Autodesk Inventor part; units mm, degrees
ref_plane "YZ Plane" through (0, 0, 0) normal (1, 0, 0) x (0, 1, 0)
ref_plane "XZ Plane" through (0, 0, 0) normal (0, 1, 0) x (-1, 0, 0)
ref_plane "XY Plane" through (0, 0, 0) normal (0, 0, 1) x (1, 0, 0)
sketch "Skizze1" plane through (0, 0, 0) normal (0, 0, 1) x (1, 0, 0)
  line L0 (15, 7.5) -> (15, -7.5)
  line L1 (15, -7.5) -> (-15, -7.5)
  line L2 (-15, -7.5) -> (-15, 7.5)
  line L3 (-15, 7.5) -> (15, -7.5) construction
  line L4 (15, 7.5) -> (-15, -7.5) construction
  arc A0 (-12.5, 7.5) -> (13.5, 7.5) centre (0.5, 7.5) ccw
  line L5 (-15, 7.5) -> (-12.5, 7.5)
  line L6 (13.5, 7.5) -> (15, 7.5)
  point P0 (0, 0)
  dimension "d0" = 30
  dimension "d1" = 15
  dimension "d2" = 26
extrude "Extrusion1" add sketch "Skizze1" along normal blind 65
sketch "Skizze2" plane through (0, 0, 65) normal (0, 0, 1) x (1, 0, 0)
  line L0 (-15, 7.5) -> (-15, -7.5)
  line L1 (15, 7.5) -> (13.5, 7.5)
  line L2 (-15, -7.5) -> (15, -7.5)
  line L3 (15, -7.5) -> (15, 7.5)
  line L4 (-15, 7.5) -> (-15, -7.5)
  arc A0 (-12.5, 7.5) -> (13.5, 7.5) centre (0.5, 7.5) ccw
  arc A1 (0, -5.4904) -> (13.5, 7.5) centre (0.5, 7.5) ccw
  arc A2 (-12.5, 7.5) -> (0, -5.4904) centre (0.5, 7.5) ccw
  point P0 (0, 0)
extrude "Extrusion2" [suppressed]
sketch "Skizze3" plane through (0, 0, 67) normal (0, 0, 1) x (1, 0, 0)
  line L0 (-15, 7.5) -> (-15, -7.5)
  line L1 (-15, -7.5) -> (15.179, -7.5)
  line L2 (15.179, -7.5) -> (15.179, 7.5)
  line L3 (15.179, 7.5) -> (-15, 7.5)
  line L4 (-15, 7.5) -> (-15, -7.5)
  arc A0 (-12.9105, 7.5) -> (13.0895, 7.5) centre (0.0895, 7.5) ccw
  point P0 (0, 0)
  dimension "d7" = 26
extrude "Extrusion3" [suppressed]
sketch "Skizze4" plane through (0, 0, 132) normal (0, 0, 1) x (1, 0, 0)
  line L0 (-15, 7.5) -> (-15, -7.5)
  line L1 (-15, -7.5) -> (15, -7.5)
  line L2 (15, -7.5) -> (15, 12.5)
  line L3 (15, 12.5) -> (-15, 12.5)
  line L4 (-15, 12.5) -> (-15, -7.5)
  point P0 (0, 0)
  dimension "d10" = 30
  dimension "d11" = 20
extrude "Extrusion4" [suppressed]
sketch "Skizze5" plane through (0, 0, 134) normal (0, 0, 1) x (1, 0, 0)
  circle A0 centre (0, 7.5) radius 2.5
  point P0 (0, 0)
  dimension "d14" = 5
extrude "Extrusion5" [suppressed]
sketch "Skizze6" plane through (0, 0, 0) normal (0, 0, -1) x (-1, 0, 0)
  line L0 (-15.179, -7.5) -> (-15, -7.5)
  line L1 (-15, 12.5) -> (15, 12.5)
  line L2 (-15, -7.5) -> (15, -7.5)
  line L3 (15, -7.5) -> (15, 12.5)
  line L4 (15, 12.5) -> (-15, 12.5)
  line L5 (-15, 12.5) -> (-15, -7.5)
  point P0 (0, 0)
  point P1 (-14.9426, -7.5)
extrude "Extrusion6" add sketch "Skizze6" along normal blind 2
sketch "Skizze7" plane through (0, 0, -2) normal (0, 0, -1) x (-1, 0, 0)
  line L0 (-13.0895, 7.5) -> (12.9105, 7.5)
  circle A0 centre (0, 7.5) radius 2.5
  point P0 (0, 0)
  dimension "d19" = 5
extrude "Extrusion7" cut sketch "Skizze7" against normal blind 2
fillet "Rundung1" radius 2 1 edges at (-15, 12.5, -1)
fillet "Rundung2" [suppressed]
fillet "Rundung3" [suppressed]
fillet "Rundung4" radius 2 1 edges at (15, 12.5, -1)
sketch "Skizze8" plane through (-15, -7.5, -2) normal (-1, 0, 0) x (0, 0, 1)
  line L0 (69, 0) -> (69, 15)
  line L1 (69, 15) -> (68, 15)
  line L2 (75.5, 13) -> (60.5, 13)
  line L3 (60.5, 13) -> (60.5, 15)
  line L4 (75.5, 15) -> (75.5, 13)
  line L5 (75.5, 13) -> (60.5, 17) construction
  line L6 (60.5, 13) -> (68, 15) construction
  line L7 (2, 15) -> (67, 15)
  line L8 (60.5, 15) -> (75.5, 15)
  point P0 (2, 7.5)
  dimension "d26" = 1
  dimension "d28" = 4
extrude "Extrusion8" add sketch "Skizze8" along normal blind 15
sketch "Skizze9" plane through (-12.5, 7.5, 65) normal (0, 1, 0) x (1, 0, 0)
  line L0 (-2.5, 6.5) -> (-17.5, 6.5)
  line L1 (-2.5, 67) -> (-2.5, 0)
  line L2 (-17.5, 6.5) -> (3.7132, 6.5) construction
  circle A0 centre (-10, -1) radius 2.5
  point P0 (12.5, 65)
  point P1 (-2.5, -69)
  dimension "d32" = 5
extrude "Extrusion9" cut sketch "Skizze9" against normal through all
sketch "Skizze10" plane through (15, -7.5, 67) normal (1, 0, 0) x (0, 0, -1)
  line L0 (0, 15) -> (1, 15)
  line L1 (67, 15) -> (2, 15)
  line L2 (8.5, 17) -> (-6.5, 17)
  line L3 (-6.5, 15) -> (-6.5, 13)
  line L4 (-6.5, 13) -> (8.5, 13)
  line L5 (8.5, 13) -> (8.5, 15)
  line L6 (1, 15) -> (-6.5, 13) construction
  line L7 (1, 15) -> (8.5, 13) construction
  line L8 (0, 15) -> (-65, 15)
  line L9 (-6.5, 15) -> (8.5, 15)
  point P0 (67, 7.5)
  point P1 (8.5, 15)
  point P2 (1, 15)
  dimension "d35" = 1
  dimension "d37" = 4
extrude "Extrusion10" add sketch "Skizze10" along normal blind 15
sketch "Skizze11" plane through (-12.5, 7.5, 65) normal (0, 1, 0) x (1, 0, 0)
  line L0 (27.679, -8.5) -> (27.679, -67)
  line L1 (42.5, -8.5) -> (42.5, 6.5)
  line L2 (27.679, -8.5) -> (48.6391, -8.5) construction
  line L3 (27.5, 6.5) -> (27.5, 0)
  circle A0 centre (35, -1) radius 2.5
  point P0 (12.5, 65)
  point P1 (27.5, -2)
  dimension "d41" = 5
extrude "Extrusion11" cut sketch "Skizze11" against normal through all
properties part number "Motorhalterung"
Design review of the part built by this model. Coordinates are the model's own, in mm. A direction names the side the tool comes from. Round coordinates to 2 decimals unless told otherwise and drop trailing zeros. Write each loop counter-clockwise with the first axis right and the second up, starting at its lowest first coordinate (ties: lowest second). Pieces come first, ordered by that corner, then holes.
Item 1: The part is to be moulded in two halves that separate along X. For faces 1 (the cylindrical face through (-14.43, 11.9, -1.01)), 2 (the flat face through (15, 7, 69)), 3 (the flat face through (20, 7.5, 59)), say which applies: +X half, -X half, draft (parallel to the pull), parting line (faces both ways), or undercut.
Item 2: We need section A-A on x = -22.5. Write out the cut boundary in (y, z), and give its area (3 significant figures).
Item 3: We need section D-D on x = 0. Write out the cut boundary in (y, z), and give its area (3 significant figures).
Item 4: We need section C-C on y = -2. Write out the cut boundary in (x, z).
Item 5: For probe 1 along X at (y, z) = (6.7, 66); probe 2 along Z at (x, y) = (22.5, 6); probe 3 along X at (y, z) = (7.5, -1.2), list the stretches that pass through material, from the lowest coordinate up.
Item 6: Clearance check with flat-ended pins moving along their axes: pin 1 Ø4.5 at (x, y) = (-3.5, -2) entering from +Z; pin 2 Ø3 at (x, y) = (0, 7.5) entering from -Z; pin 3 Ø12 at (x, z) = (-24.5, 62.5) entering from -Y; pin 4 Ø10 at (x, z) = (22, 63.5) entering from +Y. State where each tip first meets the part, or that it passes through.
Item 7: We need section B-B on z = 57.5. Write out the cut boundary in (x, y).
Item 8: For faces 4 (the flat face through (-19, 5.5, 66)), 5 (the flat face through (-22, 6, 58.5)), 6 (the flat face through (19, 5.5, 66)), 7 (the flat face through (-15, 7, 69)), list the 3-axis set-ups (+Z, -Z, +X, -X, +Y, -Y) from which the entire face can be reached by the end or side of a thin tool; tool diameter is ignored.
Returned:
1. face 1: -X half
1. face 2: undercut
1. face 3: draft
2. outline: (5.5, 58.5) - (7.5, 58.5) - (7.5, 63.5) - (5.5, 63.5) - close; (5.5, 68.5) - (7.5, 68.5) - (7.5, 73.5) - (5.5, 73.5) - close
2. area: 20.0 mm2
3. outline: (-7.5, -2) - (5, -2) - (5, 0) - (-5.49, 0) - (-5.49, 65) - (-7.5, 65) - close; (10, -2) - (12.5, -2) - (12.5, 0) - (10, 0) - close
3. area: 161 mm2
4. outline: (-15, -2) - (15, -2) - (15, 65) - (9.37, 65) - (9.37, 0) - (-8.37, 0) - (-8.37, 65) - (-15, 65) - close
5. probe 1: x = -30 to -25, -20 to -15, 15 to 20, 25 to 30
5. probe 2: z = 58.5 to 63.5, 68.5 to 73.5
5. probe 3: x = -15 to -2.5, 2.5 to 15
6. pin 1: stops at z = 0
6. pin 2: passes through
6. pin 3: stops at y = 5.5
6. pin 4: stops at y = 7.5
7. outline: (-15, -7.5) - (15, -7.5) - (15, 7.5) - (13.5, 7.5) arc R13 cw to (-12.5, 7.5) - (-15, 7.5) - close
8. face 4: +Z, -Z, -X, -Y
8. face 5: -Z, -X, +Y, -Y
8. face 6: +Z, -Z, +X, -Y
8. face 7: +Z, +Y, -Y
